For this review, take the finished solid that the model builds, in its own axes (mm). A direction names the side the tool comes from. Give positions to 0.01 mm unless a question says otherwise; leave off trailing zeros. Write each loop counter-clockwise with the first axis right and the second up, starting at its lowest first coordinate (ties: lowest second). Pieces come first, ordered by that corner, then holes. Notation, with made-up numbers: (-22, 41.5) -> (20, 41.5) arc R32 cw to (20, 74.5) -> close; hole circle Ø2 at (-13, 55.5). An arc over 180 degrees is marked (long way). Answer as CSV lines item,"result".
```python
from build123d import *

# Parameters (mm, degrees)
F0_W = 31.75
F0_H = 9.525
F2_W = 25.4
F2_H = 7.9375


# Not quite as in the source:
# - a feature names something its author has since deleted; it is built from what else it names


with BuildPart() as f1:
    # F0 (on Front) → F1 (revolve)
    with BuildSketch(Plane.XZ):
        with Locations((-41.275, 4.7625)):
            Rectangle(F0_W, F0_H)
        Polygon((-25.4, 9.525), (-25.4, 0), (-12.7, 0), (-12.7, 38.89375), (-12.7, 46.83125), (-12.7, 50.8), (-25.4, 50.8), align=None)
    revolve(axis=Axis((-41.275, 0, 0), (-1, 0, 0)))



with BuildPart() as f1b:
    # F0 (on Front) → F1, piece 2 (revolve)
    with BuildSketch(Plane.XZ):
        Polygon((12.7, 46.83125), (12.7, 38.89375), (12.7, 0), (25.4, 0), (25.4, 9.525), (25.4, 50.8), (12.7, 50.8), align=None)
    revolve(axis=Axis((-41.275, 0, 0), (-1, 0, 0)))


with BuildPart() as f1_1:
    add(f1.part)

    add(f1b.part)  # F3 merges F1b
    # F2 (on Front) → F3 (revolve)
    with BuildSketch(Plane.XZ):
        with Locations((0, 12.7)):
            Rectangle(F2_W, F2_H)
    revolve(axis=Axis((0, 0, 8.73125), (1, 0, 0)))


solid = f1_1.part
```
Q1. For faces 5 (the cylindrical face through (18.961, -49.592, -11.012)), 6 (the cylindrical face through (0.178, -2.384, 16.302)), list the 3-axis set-ups (+Z, -Z, +X, -X, +Y, -Y) from which the entire face can be reached by the end or side of a thin tool; tool diameter is ignored.
Answer block:
face 5,"+X, -X"
face 6,"none"
Q2. To check wall thickness, follow probe 1 along X at (y, z) = (6, -44); probe 2 along Z at (x, y) = (-24, 30); probe 3 along Y at (x, z) = (-20, 26.5). State the ranges of each line that lie inside material, in increasing order. Write a range as [from, to].
Answer block:
probe 1,"x = [-25.4, -12.7], [12.7, 25.4]"
probe 2,"z = [-41, 41]"
probe 3,"y = [-43.34, 43.34]"
Q3. Add section D-D (x = 16). Write out the cut boundary in (y, z).
Answer block:
outline,"circle Ø101.6 at (0, 0)"
Q4. Add section B-B (y = 0). Write out the cut boundary in (x, z) (3 decimals).
Answer block:
outline,"(-57.15, -9.525) -> (-25.4, -9.525) -> (-25.4, -50.8) -> (-12.7, -50.8) -> (-12.7, 0.794) -> (12.7, 0.794) -> (12.7, -50.8) -> (25.4, -50.8) -> (25.4, 50.8) -> (12.7, 50.8) -> (12.7, 16.669) -> (-12.7, 16.669) -> (-12.7, 50.8) -> (-25.4, 50.8) -> (-25.4, 9.525) -> (-57.15, 9.525) -> close"
Q5. Clearance check with flat-ended pins moving along their axes: pin 1 (1.5 mm diameter, centred on y = -3, z = -31.5, fed in from -X); pin 2 (5 mm diameter, centred on x = -17, z = -9, fed in from -Y); pin 3 (5 mm diameter, centred on x = -36, z = -7.5, fed in from +Y); pin 4 (4 mm diameter, centred on x = -9, y = -17, fed in from -Z). State where each tip first meets the part, or that it passes through.
Answer block:
pin 1,"stops at x = -25.4"
pin 2,"stops at y = -50.38"
pin 3,"stops at y = 8.11"
pin 4,"passes through"
Q6. Draft analysis for pull direction X (two halves, no side actions). For faces 1 (the flat face through (-25.4, 1, 11)), 2 (the cylindrical face through (-41.053, -5.796, -7.559)), 3 (the flat face through (12.7, 1, -1)), 4 (the flat face through (25.4, 1, 1)), state which applies: released by +X, released by -X, zero draft, split by the parting line, or undercut.
Answer block:
face 1,"released by -X"
face 2,"zero draft"
face 3,"undercut"
face 4,"released by +X"
Q7. Add section A-A (z = -7.5). Write out the cut boundary in (x, y).
Answer block:
outline,"(-57.15, -5.87) -> (-25.4, -5.87) -> (-25.4, -50.24) -> (-12.7, -50.24) -> (-12.7, 50.24) -> (-25.4, 50.24) -> (-25.4, 5.87) -> (-57.15, 5.87) -> close; (12.7, -50.24) -> (25.4, -50.24) -> (25.4, 50.24) -> (12.7, 50.24) -> close"
Q8. Add section C-C (y = -21.5). Write out the cut boundary in (x, z), plus the area to 3 significant figures.
Answer block:
outline,"(-25.4, -46.03) -> (-12.7, -46.03) -> (-12.7, 46.03) -> (-25.4, 46.03) -> close; (12.7, -46.03) -> (25.4, -46.03) -> (25.4, 46.03) -> (12.7, 46.03) -> close"
area,"2,340 mm2"
